Could you check a few things on this drawing? It's one solid part, dimensions in mm from its lowest x, y, z. Give positions to 0.01 mm unless a question says otherwise; leave off trailing zeros. Write each loop counter-clockwise with the first axis right and the second up, starting at its lowest first coordinate (ties: lowest second). Pieces come first, ordered by that corner, then holes. Notation, with made-up numbers: (16.5, 7) -> (51.5, 7) arc R25 cw to (51.5, 30) -> close; hole circle Ø11 at (-38, -29). An arc over 180 degrees is marked (long way). Answer as CSV lines item,"result". Start each with the question number.
1. I need wall thicknesses on line 1 (Y direction, x = 4, z = 3.25) (1 decimal); line 2 (Y direction, x = 6.5, z = 4.25) (1 decimal); line 3 (Z direction, x = 1, y = 3.75). Which ranges of each line are inside material? Lowest first, please. Write a range as [from, to].
2. If we section it at A-A on y = 21: Write out the boundary of the cut face in (x, z) (1 decimal).
3. If we section it at C-C on x = 3.5: Write out the boundary of the cut face in (y, z), plus the area to 3 significant figures.
4. I'm going to push flat-ended pins straight in: P1, Ø2.5, axis at y = 4, z = 3.847, coming from the +X side; P2, Ø3, axis at y = 16, z = 6.5, coming from the +X side; P3, Ø3, axis at y = 20, z = 2.5, coming from the +X side; P4, Ø1, axis at y = 21, z = 3.847, coming from the +X side. Where does each tip first touch, or does it pass through?
5. If we section it at D-D on z = 6.5: Write out the boundary of the cut face in (x, y).
6. If we section it at B-B on z = 3.75: Write out the boundary of the cut face in (x, y).
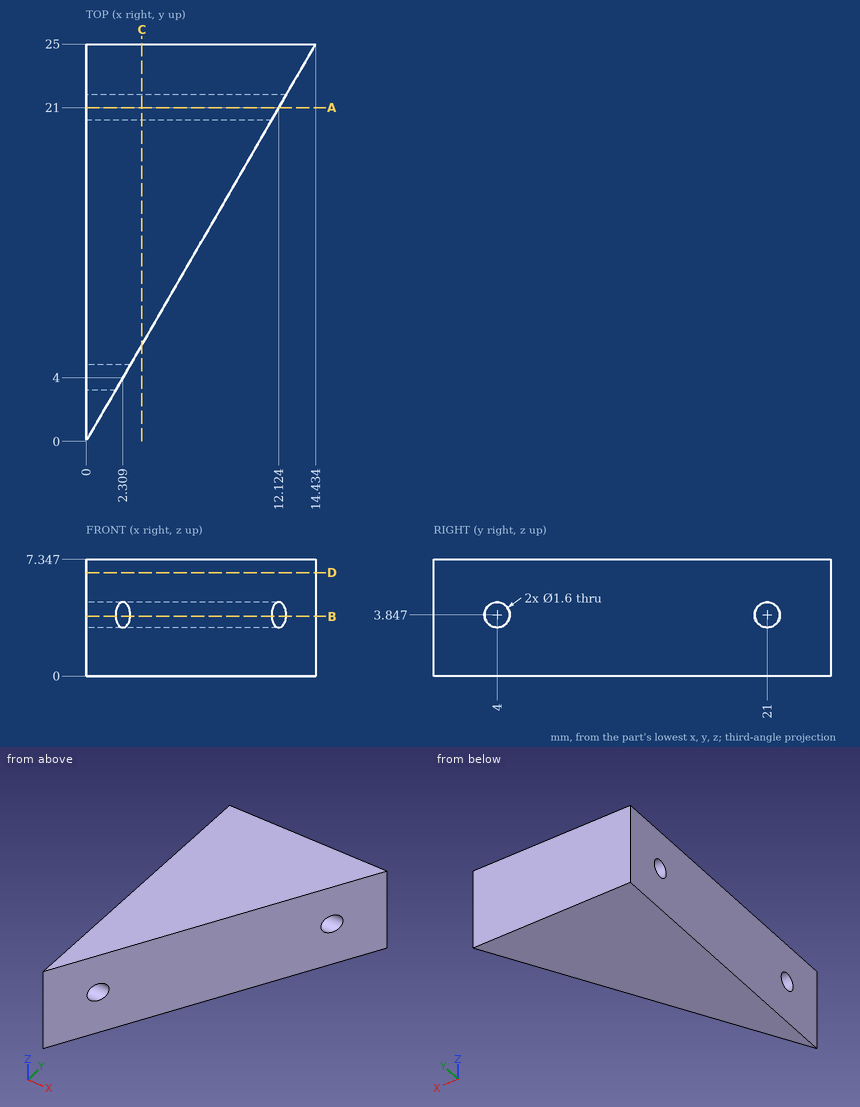
Computed values:
1,line 1,"y = [6.9, 20.5], [21.5, 25]"
1,line 2,"y = [11.3, 20.3], [21.7, 25]"
1,line 3,"z = [0, 3.09], [4.61, 7.35]"
2,outline,"(0, 0) -> (12.1, 0) -> (12.1, 3) -> (0, 3) -> close; (0, 4.6) -> (12.1, 4.6) -> (12.1, 7.3) -> (0, 7.3) -> close"
3,outline,"(6.06, 0) -> (25, 0) -> (25, 7.35) -> (6.06, 7.35) -> close; hole circle Ø1.6 at (21, 3.85)"
3,area,"137 mm2"
4,P1,"stops at x = 3.03"
4,P2,"stops at x = 10.1"
4,P3,"stops at x = 12.41"
4,P4,"passes through"
5,outline,"(0, 0) -> (14.43, 25) -> (0, 25) -> close"
6,outline,"(0, 0) -> (1.85, 3.21) -> (0, 3.21) -> close; (0, 4.79) -> (2.77, 4.79) -> (11.67, 20.21) -> (0, 20.21) -> close; (0, 21.79) -> (12.58, 21.79) -> (14.43, 25) -> (0, 25) -> close"
